Part print with two shaded views. Sizes in mm from the minimum x, y, z corner. Round coordinates to 2 decimals unless told otherwise and drop trailing zeros. Order: outer loops, then holes, each group sorted by start corner. A loop starts at its lowest first (then second) coordinate and runs counter-clockwise, first axis right, second up. Notation, with made-up numbers: (52.25, 73.25) - (68.25, 73.25) arc R13 cw to (68.25, 84.25) - close; hole circle Ø11 at (-19.5, 9.5). An arc over 180 degrees is marked (long way). Write item = value, one per line.
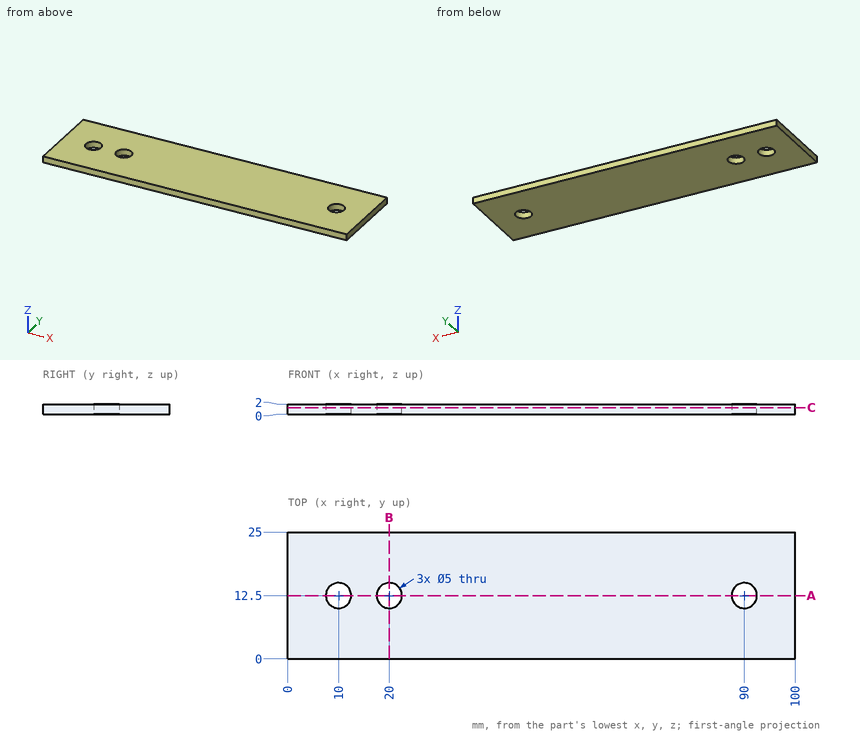
1) Cut at A-A (y = 12.5). Write the cut outline in (x, z).
Conclusion:
outline = (0, 0) - (7.5, 0) - (7.5, 2) - (0, 2) - close; (12.5, 0) - (17.5, 0) - (17.5, 2) - (12.5, 2) - close; (22.5, 0) - (87.5, 0) - (87.5, 2) - (22.5, 2) - close; (92.5, 0) - (100, 0) - (100, 2) - (92.5, 2) - close
2) Wall check: line 1 along Y through (x, z) = (20, 0.5); line 2 along Y through (x, z) = (10.5, 0.9); line 3 along X through (y, z) = (12, 0.75). Give the ranges that are in metal, low to high.
Conclusion:
line_1 = 0 to 10, 15 to 25
line_2 = 0 to 10.05, 14.95 to 25
line_3 = 0 to 7.55, 12.45 to 17.55, 22.45 to 87.55, 92.45 to 100
3) Cut at C-C (z = 1.3). Write the cut outline in (x, y), and give its area (3 significant figures).
Conclusion:
outline = (0, 0) - (100, 0) - (100, 25) - (0, 25) - close; hole circle Ø5 at (10, 12.5); hole circle Ø5 at (20, 12.5); hole circle Ø5 at (90, 12.5)
area = 2,440 mm^2
4) Flat gauge pin, fed straight in: pin 1 Ø6 at (x, y) = (20, 12.5) entering from +Z. Where does the tip first touch, or does it go through?
Conclusion:
pin_1 = 2
5) Cut at B-B (x = 20). Write the cut outline in (y, z).
Conclusion:
outline = (0, 0) - (10, 0) - (10, 2) - (0, 2) - close; (15, 0) - (25, 0) - (25, 2) - (15, 2) - close
